Input: part model. Units: mm. Frame: model coordinates. A direction names the side the tool comes from. Round coordinates to 2 decimals unless told otherwise and drop trailing zeros. Write each loop counter-clockwise with the first axis right and the second up, starting at its lowest first coordinate (ties: lowest second). Pieces come first, ordered by that corner, then holes. Notation, with made-up numbers: (-24, 20) -> (-20, 20) arc R27 cw to (-20, 45) -> close; hole circle Ø11 at (-17, 71). An arc over 180 degrees is marked (long way). Write item = value, one per line.
```python
from build123d import *

# Parameters (mm, degrees)
F0_R     = 2.2450679
F1_DEPTH = 9.525
F3_D     = 3.175
F5_D     = 3.175


# Not quite as in the source:
# - a length typed as a fraction of an inch, garbled in the dataset ("3 / 203.2 mm" for 3/8 in), is restored


with BuildPart() as f1:
    # F0 (on Top) → F1 (new body)
    with BuildSketch(Plane.XY):
        with BuildLine():
            Line((14.3843253767, 18.6275094501), (14.3843253767, 7.8833094501))
            Line((14.3843253767, 7.8833094501), (23.3759253767, 7.8833094501))
            Line((23.3759253767, 7.8833094501), (23.3759253767, 18.6275094501))
            ThreePointArc((23.3759253767, 18.6275094501), (22.0591360436, 21.806520117), (18.8801253767, 23.1233094501))
            ThreePointArc((18.8801253767, 23.1233094501), (15.7011147099, 21.806520117), (14.3843253767, 18.6275094501))
        make_face()
        with Locations((18.8801253767, 18.6275094501)):
            Circle(F0_R, mode=Mode.SUBTRACT)
        Polygon((6.1801253767, 7.8833094501), (6.1801253767, 4.7083094501), (31.5801253767, 4.7083094501), (31.5801253767, 7.8833094501), (23.3759253767, 7.8833094501), (14.3843253767, 7.8833094501), align=None)
    extrude(amount=F1_DEPTH)

    # F3 (through all)
    with Locations(Plane(origin=(0, 7.8833094501, 0), x_dir=(-1, 0, 0), z_dir=(0, 1, 0))):
        with Locations((-27.4780253767, 4.7625)):
            Hole(F3_D / 2)

    # F5 (through all)
    with Locations(Plane(origin=(0, 7.8833094501, 0), x_dir=(-1, 0, 0), z_dir=(0, 1, 0))):
        with Locations((-10.2822253767, 4.7625)):
            Hole(F5_D / 2)


solid = f1.part
```
1) Draft query along Y for faces 4 (the face through (21.022, 19.302, 4.696)), 5 (the face through (19, 4.708, 5)), 6 (the face through (28.99, 6.27, 5.24)). Return one class per face: +Y half, -Y half, draft (parallel to the pull), parting line (faces both ways), or undercut.
Solutions:
face_4 = undercut
face_5 = -Y half
face_6 = draft
2) Line query: L1, parallel to X at y = 6.5, z = 6; L2, parallel to Y at x = 13.75, z = 7; L3, parallel to X at y = 15, z = 7.5. Output: solid intervals per line, ascending. Write a range as from..to.
Solutions:
L1 = 6.18..9.29, 11.28..26.48, 28.47..31.58
L2 = 4.71..7.88
L3 = 14.38..23.38
3) Access query for faces 1 (the face through (25.7, 7.883, 4.7)), 2 (the face through (6.18, 6, 5)), 3 (the face through (12.2, 7.883, 4.7)). Directions: +Z, -Z, +X, -X, +Y, -Y. A direction counts if a zero-diameter tool reaches every point of the face in a straight line with its end or side. Return the directions, or none.
Solutions:
face_1 = +Z, -Z, +X, +Y
face_2 = +Z, -Z, -X, +Y, -Y
face_3 = +Z, -Z, -X, +Y
4) Cut plane B-B (y = 18). Return the cut outline in (x, z) (3 decimals), and give its area (3 significant figures).
Solutions:
outline = (14.384, 0) -> (16.725, 0) -> (16.725, 9.525) -> (14.384, 9.525) -> close; (21.036, 0) -> (23.376, 0) -> (23.376, 9.525) -> (21.036, 9.525) -> close
area = 44.6 mm^2
5) Cut plane C-C (x = 19.75). Return the cut outline in (y, z) (3 decimals), and give its area (3 significant figures).
Solutions:
outline = (4.708, 0) -> (16.558, 0) -> (16.558, 9.525) -> (4.708, 9.525) -> close; (20.697, 0) -> (23.038, 0) -> (23.038, 9.525) -> (20.697, 9.525) -> close
area = 135 mm^2
6) Cut plane A-A (z = 7.25). Return the cut outline in (x, y).
Solutions:
outline = (6.18, 4.71) -> (31.58, 4.71) -> (31.58, 7.88) -> (23.38, 7.88) -> (23.38, 18.63) arc R4.5 ccw to (14.38, 18.63) -> (14.38, 7.88) -> (6.18, 7.88) -> close; hole circle Ø4.49 at (18.88, 18.63)
7) Cut plane D-D (z = 4.5). Return the cut outline in (x, y).
Solutions:
outline = (6.18, 4.71) -> (8.72, 4.71) -> (8.72, 7.88) -> (6.18, 7.88) -> close; (11.85, 4.71) -> (25.91, 4.71) -> (25.91, 7.88) -> (23.38, 7.88) -> (23.38, 18.63) arc R4.5 ccw to (14.38, 18.63) -> (14.38, 7.88) -> (11.85, 7.88) -> close; (29.04, 4.71) -> (31.58, 4.71) -> (31.58, 7.88) -> (29.04, 7.88) -> close; hole circle Ø4.49 at (18.88, 18.63)
8) First-contact query: P1, Ø4, axis at y = 17.5, z = 2, coming from the -X side; P2, Ø3.5, axis at x = 10.28, z = 4.76, coming from the +Y side. Flat tips, straight axial feed; report the tip coordinate or a pass-through.
Solutions:
P1 = 14.38
P2 = 7.88
